Input: part model. Units: mm. Frame: model coordinates. Coordinates: 2 decimals unless noted, no trailing zeros. Write each loop counter-clockwise with the first axis right and the second up, starting at its lowest first coordinate (ties: lowest second). Pieces come first, ordered by that corner, then holes.
1) Line query: L1, parallel to X at y = 64.5, z = -299.5; L2, parallel to Y at x = -25.5, z = -342; L3, parallel to Z at x = -263, y = 232.5. Output: solid intervals per line, ascending.
2) Draft query along X for faces 1 (the flat face through (-5, 185, -675)), 2 (the flat face through (-337.5, 185, -333)), 3 (the flat face through (335, 184, -332)), 4 (the flat face through (337.5, 185, -333)). Return one class per face: pulls with the +X half, pulls with the -X half, needs draft (parallel to the pull), parting line crosses it, or undercut.
3) Section query A-A (y = 306). Output: boundary loops of the cut face in (x, z), then the cut area to 3 significant figures.
4) Pin query (flat end, axial travel): pin 1 Ø5 at (x, z) = (6, -7) entering from -Y; pin 2 Ø8 at (x, z) = (264.5, -589) entering from -Y; pin 3 Ø5 at (x, y) = (171, 45.5) entering from +Z. Return the tip coordinate at first contact, or that it passes through.
5) Section query C-C (z = -155.5). Output: boundary loops of the cut face in (x, y).
6) Section query B-B (x = -220.5). Output: boundary loops of the cut face in (y, z), then the cut area to 4 significant figures.
from build123d import *

# Parameters (mm, degrees)
SKETCH1_W           = 675
SKETCH1_H           = 675
BOSS_EXTRUDE1_DEPTH = 375
CUT_EXTRUDE3_START  = -10
SKETCH4_W           = 670
SKETCH4_H           = 370
CUT_EXTRUDE3_DEPTH  = 662.5
SKETCH6_W           = 670
SKETCH6_H           = 5
CUT_EXTRUDE4_DEPTH  = 670
SKETCH11_W          = 213.34
SKETCH11_H          = 360
SKETCH11_W_2        = 213.33
CUT_EXTRUDE6_DEPTH  = 10


with BuildPart() as part:
    # Sketch1 → Boss-Extrude1 (new body)
    with BuildSketch(Plane(origin=(0, 0, 0), x_dir=(1, 0, 0), z_dir=(0, 1, 0))):
        with Locations((0, 337.5)):
            Rectangle(SKETCH1_W, SKETCH1_H)
    extrude(amount=BOSS_EXTRUDE1_DEPTH)

    # Sketch4 → Cut-Extrude3 (cut)
    with BuildSketch(Plane.XY.offset(CUT_EXTRUDE3_START)):
        with Locations((0, 187.5)):
            Rectangle(SKETCH4_W, SKETCH4_H)
    extrude(amount=-CUT_EXTRUDE3_DEPTH, mode=Mode.SUBTRACT)

    # Sketch6 → Cut-Extrude4 (cut)
    with BuildSketch(Plane.XY):
        Rectangle(SKETCH6_W, SKETCH6_H)
    extrude(amount=-CUT_EXTRUDE4_DEPTH, mode=Mode.SUBTRACT)

    # Sketch11 → Cut-Extrude6 (cut)
    with BuildSketch(Plane.XY):
        with Locations((0, 187.5)):
            Rectangle(SKETCH11_W, SKETCH11_H)
        with Locations((-220.835, 187.5)):
            Rectangle(SKETCH11_W_2, SKETCH11_H)
        with Locations((220.835, 187.5)):
            Rectangle(SKETCH11_W_2, SKETCH11_H)
    extrude(amount=-CUT_EXTRUDE6_DEPTH, mode=Mode.SUBTRACT)


solid = part.part
Answer:
1. L1: x = -337.5 to -335, 335 to 337.5
1. L2: y = 372.5 to 375
1. L3: z = -675 to -672.5
2. face 1: needs draft
2. face 2: pulls with the -X half
2. face 3: undercut
2. face 4: pulls with the +X half
3. outline: (-337.5, -675) - (337.5, -675) - (337.5, 0) - (327.5, 0) - (327.5, -10) - (335, -10) - (335, -672.5) - (-335, -672.5) - (-335, -10) - (-327.5, -10) - (-327.5, 0) - (-337.5, 0) - close; (-114.17, -10) - (-106.67, -10) - (-106.67, 0) - (-114.17, 0) - close; (106.67, -10) - (114.17, -10) - (114.17, 0) - (106.67, 0) - close
3. area: 5,350 mm2
4. pin 1: stops at y = 2.5
4. pin 2: stops at y = 372.5
4. pin 3: stops at z = -672.5
5. outline: (-337.5, 0) - (-335, 0) - (-335, 372.5) - (335, 372.5) - (335, 0) - (337.5, 0) - (337.5, 375) - (-337.5, 375) - close
6. outline: (0, -675) - (375, -675) - (375, 0) - (367.5, 0) - (367.5, -10) - (372.5, -10) - (372.5, -672.5) - (2.5, -672.5) - (2.5, -670) - (0, -670) - close; (2.5, -10) - (7.5, -10) - (7.5, 0) - (2.5, 0) - close
6. area: 2,725 mm2
